Geometry check sheet. Reference: the model listing, model coordinates, mm. A direction names the side the tool comes from. Round coordinates to 2 decimals unless told otherwise and drop trailing zeros. Write each loop counter-clockwise with the first axis right and the second up, starting at its lowest first coordinate (ties: lowest second). Pieces come first, ordered by that corner, then holes. Notation, with made-up numbers: (-28, -10) -> (26, -10) arc R9 ccw to (26, 7) -> close; hole circle Ø6 at (87.25, 56). An arc over 180 degrees is marked (long way). Return JSON: item names as keys, results as strings. Group by question number.
from build123d import *

# Parameters (mm, degrees)
BOSS_EXTRUDE1_DEPTH = 5
SKETCH2_R           = 1.75
CUT_EXTRUDE1_DEPTH  = 93.552687697
SKETCH3_R           = 4
CUT_EXTRUDE2_DEPTH  = 93.552687697
SKETCH4_R           = 5
CUT_EXTRUDE3_DEPTH  = 93.552687697
SKETCH6_R           = 6
SKETCH6_R_2         = 4
BOSS_EXTRUDE3_DEPTH = 1


with BuildPart() as part:
    # Sketch1 → Boss-Extrude1 (new body)
    with BuildSketch(Plane.XY):
        with BuildLine():
            Line((-21, 0), (-21, 90))
            Line((-21, 90), (21, 90))
            Line((21, 90), (21, 0))
            ThreePointArc((21, 0), (0, -21), (-21, 0))
        make_face()
    extrude(amount=BOSS_EXTRUDE1_DEPTH)

    # Sketch2 → Cut-Extrude1 (cut, through all)
    with BuildSketch(Plane(origin=(0, 0, 0), x_dir=(-1, 0, 0), z_dir=(0, 0, -1))):
        with Locations((-15, 85)):
            Circle(SKETCH2_R)
        with Locations((-15, 64)):
            Circle(SKETCH2_R)
        with Locations(Location((15, 64, 0), (0, 0, 180))):
            Circle(SKETCH2_R)
        with Locations(Location((15, 85, 0), (0, 0, 180))):
            Circle(SKETCH2_R)
    extrude(amount=-CUT_EXTRUDE1_DEPTH, mode=Mode.SUBTRACT)

    # Sketch3 → Cut-Extrude2 (cut, through all)
    with BuildSketch(Plane(origin=(0, 0, 0), x_dir=(-1, 0, 0), z_dir=(0, 0, -1))):
        Circle(SKETCH3_R)
    extrude(amount=-CUT_EXTRUDE2_DEPTH, mode=Mode.SUBTRACT)

    # Sketch4 → Cut-Extrude3 (cut, through all)
    with BuildSketch(Plane(origin=(0, 0, 0), x_dir=(-1, 0, 0), z_dir=(0, 0, -1))):
        with Locations((0, 28)):
            Circle(SKETCH4_R)
    extrude(amount=-CUT_EXTRUDE3_DEPTH, mode=Mode.SUBTRACT)

    # Sketch6 → Boss-Extrude3 (add)
    with BuildSketch(Plane.XY.offset(5)):
        Circle(SKETCH6_R)
        with Locations(Location((0, 0, 0), (0, 0, 180))):
            Circle(SKETCH6_R_2, mode=Mode.SUBTRACT)
    extrude(amount=BOSS_EXTRUDE3_DEPTH)


solid = part.part
1) Tool access check on faces 4 (the face through (-15.38, 86.71, 2.46)), 5 (the face through (-5.994, 0.264, 5.493)). Record the directions out of +Z, -Z, +X, -X, +Y, -Y that give a thin tool (end or side, any length) a straight path to the whole face; none if there is none.
2) Go/stop test with flat-tipped pins: P1, Ø1.5, axis at x = -5, z = 5.5, coming from the -Y side; P2, Ø4, axis at x = -15, y = 85, coming from the +Z side; P3, Ø6, axis at x = 0, y = 28, coming from the +Z side; P4, Ø2, axis at x = -2, z = 2.5, coming from the -Y side. Record where each tip stops, or that it passes through.
3) Sectioned sample at C-C on z = 2.8. Enter the section's corners in (x, y).
4) Sectioned sample at A-A on x = 0. Enter the section's corners in (y, z).
5) Mould release check, pull along X, two halves, no side actions. Record for faces 1 (the face through (0, -21, 2)), 2 (the face through (1.08, 23.12, 2.46)), 3 (the face through (0, 35, 5)): +X half, -X half, draft (parallel to the pull), parting line (faces both ways), or undercut.
6) Material ranges on probe 1 along X at (y, z) = (64, 3.05); probe 2 along Y at (x, z) = (0, 2.65); probe 3 along Y at (x, z) = (15, 1.4), recorded low to high. Write a range as [from, to].
7) Sectioned sample at B-B on y = 28. Enter the section's corners in (x, z).
8) Sectioned sample at D-D on y = 85. Enter the section's corners in (x, z), and give its area (3 significant figures).
Evaluation:
{
 "1": {"face 4": "+Z, -Z", "face 5": "+Z"},
 "2": {"P1": "stops at y = -20.53", "P2": "stops at z = 5", "P3": "passes through", "P4": "stops at y = -20.98"},
 "3": {"outline": "(-21, 0) arc R21 ccw to (21, 0) -> (21, 90) -> (-21, 90) -> close; hole circle Ø3.5 at (-15, 64); hole circle Ø3.5 at (-15, 85); hole circle Ø10 at (0, 28); hole circle Ø8 at (0, 0); hole circle Ø3.5 at (15, 64); hole circle Ø3.5 at (15, 85)"},
 "4": {"outline": "(-21, 0) -> (-4, 0) -> (-4, 6) -> (-6, 6) -> (-6, 5) -> (-21, 5) -> close; (4, 0) -> (23, 0) -> (23, 5) -> (6, 5) -> (6, 6) -> (4, 6) -> close; (33, 0) -> (90, 0) -> (90, 5) -> (33, 5) -> close"},
 "5": {"face 1": "parting line", "face 2": "undercut", "face 3": "draft"},
 "6": {"probe 1": "x = [-21, -16.75], [-13.25, 13.25], [16.75, 21]", "probe 2": "y = [-21, -4], [4, 23], [33, 90]", "probe 3": "y = [-14.7, 62.25], [65.75, 83.25], [86.75, 90]"},
 "7": {"outline": "(-21, 0) -> (-5, 0) -> (-5, 5) -> (-21, 5) -> close; (5, 0) -> (21, 0) -> (21, 5) -> (5, 5) -> close"},
 "8": {"outline": "(-21, 0) -> (-16.75, 0) -> (-16.75, 5) -> (-21, 5) -> close; (-13.25, 0) -> (13.25, 0) -> (13.25, 5) -> (-13.25, 5) -> close; (16.75, 0) -> (21, 0) -> (21, 5) -> (16.75, 5) -> close", "area": "175 mm2"}
}
